Here's how the part is built. I have some questions about the finished solid (model axes, mm). Face numbers are marked on the shaded views. Coordinates: 2 decimals unless noted, no trailing zeros. Loops run counter-clockwise (first coordinate to the right, second up) from the corner with the lowest first, then second, coordinate; pieces in that order, holes last. Notation, with made-up numbers: M 60,66 L 101,66 A21 ccw 101,82 Z; hole C -24.5,18 d4. An arc over 180 degrees is marked long. Use one line per item in the form item = value. Start each with the question number.
(1) Imagine slicing it at C-C, the plane z = 514.5. Please give me the cut outline in (x, y).
(2) Will these pins go through, and if not, where does the flat tip stop? P1, Ø4, axis at y = -59, z = 189.5, coming from the -X side; P2, Ø8, axis at x = -88, z = 342.5, coming from the -Y side; P3, Ø4, axis at x = -64.5, z = 748.5, coming from the -Y side.
(3) Thinking about a two-plate mould opening in Z: for the marked faces 1, 2 and 3, which applies, +Z half, -Z half, draft (parallel to the pull), parting line (faces both ways), or undercut?
(4) Imagine slicing it at A-A, the plane y = 0. Please give me the cut outline in (x, z), and give its area (3 significant figures).
(5) Please list where these lines run through material, in increasing order: L1, parallel to Z at x = 77, y = -350; L2, parallel to Y at x = 0, z = 779.5; L3, parallel to X at y = -118, z = 709.
(6) Imagine slicing it at D-D, the plane x = 326.5. Please give me the cut outline in (y, z).
```python
from build123d import *

# Parameters (mm, degrees)
SKETCH2_R           = 200
BOSS_EXTRUDE1_DEPTH = 1000
SKETCH3_R           = 600
BOSS_EXTRUDE2_DEPTH = 50
BOSS_EXTRUDE3_START = 50
SKETCH4_R           = 600
BOSS_EXTRUDE3_DEPTH = 50
SKETCH5_R           = 50
CUT_EXTRUDE1_DEPTH  = 1390.244398945


with BuildPart() as part:
    # Sketch2 → Boss-Extrude1 (new body)
    with BuildSketch(Plane.XY):
        Circle(SKETCH2_R)
    extrude(amount=BOSS_EXTRUDE1_DEPTH)

    # Sketch3 → Boss-Extrude2 (add)
    with BuildSketch(Plane.XY.offset(1000)):
        Circle(SKETCH3_R)
    extrude(amount=BOSS_EXTRUDE2_DEPTH)

    # Sketch4 → Boss-Extrude3 (add)
    with BuildSketch(Plane(origin=(0, 0, 0), x_dir=(-1, 0, 0), z_dir=(0, 0, -1)).offset(BOSS_EXTRUDE3_START)):
        with Locations(Location((0, 0, 0), (0, 0, 180))):
            Circle(SKETCH4_R)
    extrude(amount=-BOSS_EXTRUDE3_DEPTH)

    # Sketch5 → Cut-Extrude1 (cut, through all)
    with BuildSketch(Plane.XY.offset(1050)):
        Circle(SKETCH5_R)
    extrude(amount=-CUT_EXTRUDE1_DEPTH, mode=Mode.SUBTRACT)


solid = part.part
```
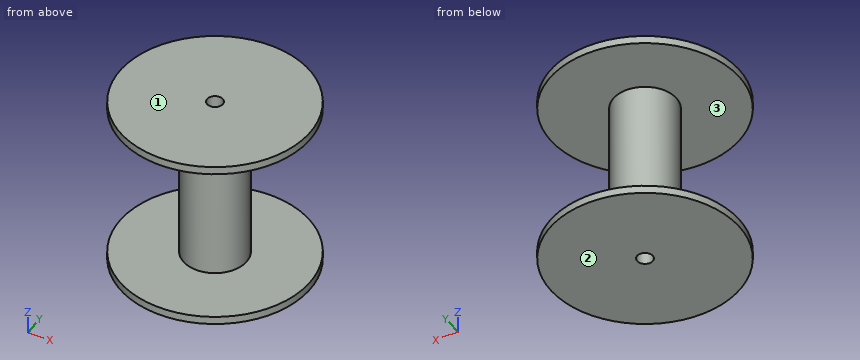
Answer:
q1.outline = C 0,0 d400; hole C 0,0 d100
q2.P1 = -191.71
q2.P2 = -181.5
q2.P3 = -189.98
q3.face_1 = +Z half
q3.face_2 = -Z half
q3.face_3 = undercut
q4.outline = M -600,-50 L -50,-50 L -50,1050 L -600,1050 L -600,1000 L -200,1000 L -200,0 L -600,0 Z; M 50,-50 L 600,-50 L 600,0 L 200,0 L 200,1000 L 600,1000 L 600,1050 L 50,1050 Z
q4.area = 410,000 mm²
q5.L1 = -50 to 0, 1000 to 1050
q5.L2 = -200 to -50, 50 to 200
q5.L3 = -161.48 to 161.48
q6.outline = M -503.39,-50 L 503.39,-50 L 503.39,0 L -503.39,0 Z; M -503.39,1000 L 503.39,1000 L 503.39,1050 L -503.39,1050 Z
